Can you work these out from the model? Positions are in its coordinate system, mm. Coordinates: 2 decimals unless noted, no trailing zeros. Order: outer loops, then holes, each group sorted by start corner. A loop starts at its lowest first (then second) coordinate and runs counter-clockwise, first axis right, second up. Notation, with made-up numbers: (21, 83) - (78, 83) arc R18 ccw to (78, 98) - close; hole circle Ø10 at (-24.75, 66.25). An arc over 180 degrees is marked (long way). Use a Markdown table: item, result. Add a question column.
(1) I want a section at C-C (z = 35). List the corners of the cut face in (x, y) for me.
(2) I want a section at A-A (y = -0.85). List the corners of the cut face in (x, z) for me.
(3) If I drill on L1, parallel to Z at x = 35, y = 0.1; L2, parallel to X at y = 0.35, z = 35; L3, parallel to Z at x = -34, y = -0.75, over which ranges is the centre line in solid material (lowest first)? Write a range as [from, to].
(4) I want a section at D-D (x = 6). List the corners of the cut face in (y, z) for me, and give its area (3 significant figures).
(5) I want a section at B-B (x = 35). List the corners of the cut face in (y, z) for me, and give its area (3 significant figures).
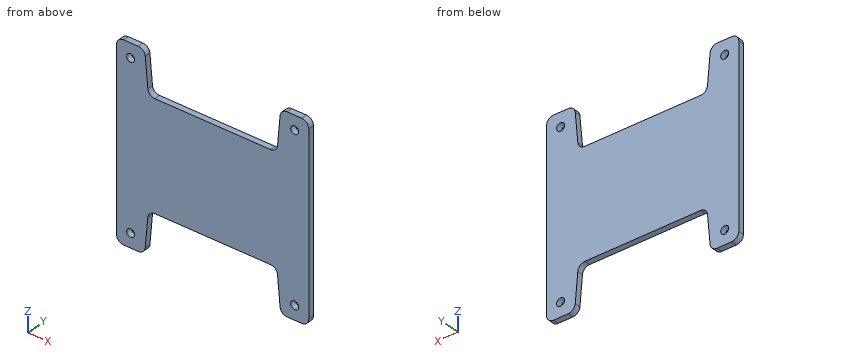
```python
from build123d import *

# Parameters (mm, degrees)
SKETCH1_W            = 82
SKETCH1_H            = 82
BOSS_EXTRUDE1_DEPTH  = 1.25
M3_CLEARANCE_HOLE1_D = 3.4
CUT_EXTRUDE1_DEPTH   = 59.036626366
FILLET1_R            = 3


with BuildPart() as part:
    # Sketch1 → Boss-Extrude1 (new, symmetric)
    with BuildSketch(Plane(origin=(0, 0, 0), x_dir=(1, 0, 0), z_dir=(0, 1, 0))):
        Rectangle(SKETCH1_W, SKETCH1_H)
    extrude(amount=BOSS_EXTRUDE1_DEPTH, both=True)

    # M3 Clearance Hole1 (through all)
    with Locations(Plane(origin=(0, 1.25, 0), x_dir=(1, 0, 0), z_dir=(0, 1, 0))):
        with Locations((35, 35), (-35, -35), (-35, 35), (35, -35)):
            Hole(M3_CLEARANCE_HOLE1_D / 2)

    # Sketch4 → Cut-Extrude1 (cut, through all)
    with BuildSketch(Plane(origin=(0, -1.25, 0), x_dir=(-1, 0, 0), z_dir=(0, -1, 0))):
        Polygon((-29, -41), (29, -41), (27.425204057, -23), (-27.425204057, -23), align=None)
        Polygon((29, 41), (-29, 41), (-27.425204057, 23), (0, 23), (27.425204057, 23), align=None)
    extrude(amount=-CUT_EXTRUDE1_DEPTH, mode=Mode.SUBTRACT)

    # Fillet1
    fillet1_edges = [part.edges().sort_by_distance(p)[0] for p in [
        (29, 0, 41),
        (27.425204057, 0, 23),
        (-27.425204057, 0, 23),
        (-29, 0, 41),
        (-29, 0, -41),
        (-27.425204057, 0, -23),
        (27.425204057, 0, -23),
        (29, 0, -41),
        (-41, 0, -41),
        (41, 0, -41),
        (41, 0, 41),
        (-41, 0, 41),
    ]]
    fillet(fillet1_edges, radius=FILLET1_R)


solid = part.part
```
Answers follow:
| question | item | result |
|---|---|---|
| 1 | outline | (-41, -1.25) - (-36.7, -1.25) - (-36.7, 1.25) - (-41, 1.25) - close; (-33.3, -1.25) - (-28.48, -1.25) - (-28.48, 1.25) - (-33.3, 1.25) - close; (28.48, -1.25) - (33.3, -1.25) - (33.3, 1.25) - (28.48, 1.25) - close; (36.7, -1.25) - (41, -1.25) - (41, 1.25) - (36.7, 1.25) - close |
| 2 | outline | (-41, -38) arc R3 ccw to (-38, -41) - (-31.75, -41) arc R3 ccw to (-28.76, -38.26) - (-27.66, -25.74) arc R3 cw to (-24.68, -23) - (24.68, -23) arc R3 cw to (27.66, -25.74) - (28.76, -38.26) arc R3 ccw to (31.75, -41) - (38, -41) arc R3 ccw to (41, -38) - (41, 38) arc R3 ccw to (38, 41) - (31.75, 41) arc R3 ccw to (28.76, 38.26) - (27.66, 25.74) arc R3 cw to (24.68, 23) - (-24.68, 23) arc R3 cw to (-27.66, 25.74) - (-28.76, 38.26) arc R3 ccw to (-31.75, 41) - (-38, 41) arc R3 ccw to (-41, 38) - close; hole circle Ø3.4 at (-35, -35); hole circle Ø3.4 at (-35, 35); hole circle Ø3.4 at (35, -35); hole circle Ø3.4 at (35, 35) |
| 3 | L1 | z = [-41, -36.7], [-33.3, 33.3], [36.7, 41] |
| 3 | L2 | x = [-41, -36.7], [-33.3, -28.48], [28.48, 33.3], [36.7, 41] |
| 3 | L3 | z = [-41, -36.37], [-33.63, 33.63], [36.37, 41] |
| 4 | outline | (-1.25, -23) - (1.25, -23) - (1.25, 23) - (-1.25, 23) - close |
| 4 | area | 115 mm² |
| 5 | outline | (-1.25, -41) - (1.25, -41) - (1.25, -36.7) - (-1.25, -36.7) - close; (-1.25, -33.3) - (1.25, -33.3) - (1.25, 33.3) - (-1.25, 33.3) - close; (-1.25, 36.7) - (1.25, 36.7) - (1.25, 41) - (-1.25, 41) - close |
| 5 | area | 188 mm² |
